Geometry: final body of the model. Coordinates: model frame, mm. Face numbers are marked on the shaded views. Give positions to 0.01 mm unless a question says otherwise; leave off trailing zeros. Write each loop counter-clockwise with the first axis right and the second up, starting at its lowest first coordinate (ties: lowest second). Pieces come first, ordered by that corner, then holes. Notation, with made-up numbers: (72.5, -26.75) -> (120.5, -26.75) arc R16 ccw to (120.5, 1.25) -> close; hole circle Ø5 at (88, -15.75). An arc over 180 degrees is marked (long way). Answer in a Markdown table with one row per item. Add a question column.
from build123d import *

# Parameters (mm, degrees)
SKETCH1_R           = 4
BOSS_EXTRUDE1_DEPTH = 40
CUT_EXTRUDE1_START  = -2.5
CUT_EXTRUDE1_DEPTH  = 2.5
SKETCH3_W           = 0.6
SKETCH3_H           = 2.558346845
BOSS_EXTRUDE2_DEPTH = 10
CIRPATTERN1_COUNT   = 10
CHAMFER1_SIZE       = 0.5


with BuildPart() as part:
    # Sketch1 → Boss-Extrude1 (new body)
    with BuildSketch(Plane.XY):
        Circle(SKETCH1_R)
    extrude(amount=BOSS_EXTRUDE1_DEPTH)

    # Sketch2 → Cut-Extrude1 (cut, through all)
    with BuildSketch(Plane(origin=(0, 0, 0), x_dir=(1, 0, 0), z_dir=(0, 1, 0)).offset(CUT_EXTRUDE1_START)):
        with BuildLine():
            Line((1.5, -5), (1.5, -9))
            ThreePointArc((1.5, -9), (0, -10.5), (-1.5, -9))
            Line((-1.5, -9), (-1.5, -5))
            ThreePointArc((-1.5, -5), (0, -3.5), (1.5, -5))
        make_face()
    extrude(amount=-CUT_EXTRUDE1_DEPTH, mode=Mode.SUBTRACT)

    # Sketch3 → Boss-Extrude2 (add)
    with BuildSketch(Plane.XY.offset(40)):
        with Locations((0, 3.220826578)):
            Rectangle(SKETCH3_W, SKETCH3_H)
    boss_extrude2 = extrude(amount=-BOSS_EXTRUDE2_DEPTH)

    # CirPattern1: Boss-Extrude2 ×10 about axis
    cirpattern1_axis = Axis((0, 0, 0), (0, 0, 1))
    for i in range(1, CIRPATTERN1_COUNT):
        add(boss_extrude2.rotate(cirpattern1_axis, i * 360 / CIRPATTERN1_COUNT))

    # Chamfer1
    chamfer1_edges = [part.edges().sort_by_distance(p)[0] for p in [
        (-4, 0, 0),
    ]]
    chamfer(chamfer1_edges, length=CHAMFER1_SIZE)


solid = part.part
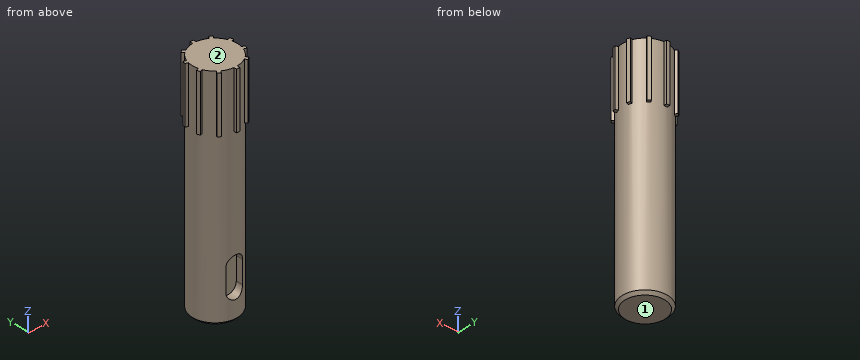
Q1. Contact query for flat-ended pins moving along their axis: pin 1 Ø4 at (x, z) = (2.5, 6) entering from +Y; pin 2 Ø1.3 at (y, z) = (-3.5, 7.5) entering from +X; pin 3 Ø5 at (x, z) = (2, 33.5) entering from -Y; pin 4 Ø0.6 at (y, z) = (-3.5, 7) entering from -X. Output: stop coordinate, or through.
Q2. Pull-direction query (Z, two-part tool) for the marked faces 1 and 2; classes: +Z half, -Z half, draft (parallel to the pull), parting line (faces both ways), or undercut.
Q3. Line query: probe 1 along Y at (x, z) = (-1.5, 25.5); probe 2 along X at (y, z) = (-2, 23.5). Output: solid intervals per line, ascending. Write a range as from..to.
Q4. Section A-A on y = 0. Return loops of the section in (x, z).
Q5. Section B-B on z = 15. Return loops of the section in (x, y), and give its area (3 significant figures).
Checks:
| question | item | result |
|---|---|---|
| 1 | pin 1 | y = 3.97 |
| 1 | pin 2 | x = 2.81 |
| 1 | pin 3 | y = -4.5 |
| 1 | pin 4 | x = -2.4 |
| 2 | face 1 | -Z half |
| 2 | face 2 | +Z half |
| 3 | probe 1 | -3.71..3.71 |
| 3 | probe 2 | -3.46..3.46 |
| 4 | outline | (-4, 0.5) -> (-3.5, 0) -> (3.5, 0) -> (4, 0.5) -> (4, 40) -> (-4, 40) -> close |
| 5 | outline | circle Ø8 at (0, 0) |
| 5 | area | 50.3 mm^2 |
